For this review, take the finished solid that the model builds, in its own axes (mm). Coordinates: 2 decimals unless noted, no trailing zeros. Write each loop counter-clockwise with the first axis right and the second up, starting at its lowest first coordinate (ties: lowest second). Pieces come first, ordered by that corner, then holes. Notation, with made-up numbers: (60.5, 27) - (68.5, 27) arc R16 cw to (68.5, 48) - close; hole circle Ø3 at (46, 3.25). An arc over 180 degrees is marked (long way). Use one line per item in the form item = value. Start each with the question number.
1) We need section A-A (z = 3.25). Give the boundary of the cut face in (x, y).
2) Mouldability with a two-part tool opening along Y and no side actions: class faces 1 (the flat face through (-42, 0, 6.35)), 2 (the flat face through (-44, -3.969, 3)), 3 (the flat face through (-42, 3.969, 3)), 4 (the cylindrical face through (-30.36, -0.86, 3.13)) as pulls with the +Y half, pulls with the -Y half, needs draft (parallel to the pull), parting line crosses it, or undercut.
3) For L1, parallel to X at y = 1.25, z = 3.75; L2, parallel to X at y = 0.75, z = 3; L3, parallel to X at y = 2.5, z = 2, list the stretches that pass through material, from the lowest coordinate up. Write a range as from..to.
4) Insertion check: P1, Ø3.5, axis at x = -32.44, y = 0, coming from the +Z side; P2, Ø3, axis at y = -1, z = 2.5, coming from the +X side. Each pin has a flat end and moves straight along its axis. Give the tip position at first contact, or say it passes through.
```python
from build123d import *

# Parameters (mm, degrees)
F0_R     = 2.2479
F1_DEPTH = 6.35


with BuildPart() as f1:
    # F0 (on Top) → F1 (new body)
    with BuildSketch(Plane.XY):
        with BuildLine():
            ThreePointArc((0, 2.2479), (1.589505, 1.589505), (2.2479, 0))
            ThreePointArc((2.2479, 0), (1.589505, -1.589505), (0, -2.2479))
            Line((0, -2.2479), (0, -3.96875))
            ThreePointArc((0, -3.96875), (3.96875, 0), (0, 3.96875))
            Line((0, 3.96875), (0, 2.2479))
        make_face()
        with BuildLine():
            ThreePointArc((0, -2.2479), (-2.2479, 0), (0, 2.2479))
            Line((0, 2.2479), (0, 3.96875))
            Line((0, 3.96875), (-86.148189, 3.96875))
            Line((-86.148189, 3.96875), (-86.148189, -3.96875))
            Line((-86.148189, -3.96875), (0, -3.96875))
            Line((0, -3.96875), (0, -2.2479))
        make_face()
        with Locations((-32.438553, 0)):
            Circle(F0_R, mode=Mode.SUBTRACT)
    extrude(amount=F1_DEPTH)


solid = f1.part
```
Determined:
q1.outline = (-86.15, -3.97) - (0, -3.97) arc R3.97 ccw to (0, 3.97) - (-86.15, 3.97) - close; hole circle Ø4.5 at (-32.44, 0); hole (0, -2.25) arc R2.25 ccw to (2.25, 0) arc R2.25 ccw to (0, 2.25) arc R2.25 ccw to start
q2.face_1 = needs draft
q2.face_2 = pulls with the -Y half
q2.face_3 = pulls with the +Y half
q2.face_4 = undercut
q3.L1 = -86.15..-34.31, -30.57..-1.87, 1.87..3.77
q3.L2 = -86.15..-34.56, -30.32..-2.12, 2.12..3.9
q3.L3 = -86.15..3.08
q4.P1 = through
q4.P2 = 3.97
